Design review of the part built by this model. Coordinates are the model's own, in mm. A direction names the side the tool comes from. Coordinates: 2 decimals unless noted, no trailing zeros. Loops run counter-clockwise (first coordinate to the right, second up) from the corner with the lowest first, then second, coordinate; pieces in that order, holes last. Notation, with made-up numbers: M -4.75,17.5 L 16.25,17.5 A6 cw 16.25,28.5 Z; hole C 73,7.5 d8. An arc over 180 degrees is marked long. Answer as a JSON object with one key per item and string values. Group by question number.
1. Consider section B-B (x = 0). State the section outline as (y, z) points, then the cut area to 3 significant figures.
2. Consider section C-C (z = 0.5). State the section outline as (x, y) points, then the cut area to 3 significant figures.
3. Draft analysis for pull direction Y (two halves, no side actions). For faces 1 (the cylindrical face through (-0.867, -3.905, 4.085)), 2 (the flat face through (0, 0, 0)), 3 (the flat face through (1.748, 0.986, 6.028)), state which applies: +Y half, -Y half, draft (parallel to the pull), parting line (faces both ways), or undercut.
4. Insertion check: pin 1 (0.6 mm diameter, centred on x = 0.5, z = 5.5, fed in from -Y) (3 decimals); pin 2 (2 mm diameter, centred on x = 3, z = 6.5, fed in from -Y); pin 3 (4 mm diameter, centred on x = 2.5, z = 2.5, fed in from +Y). Each pin has a flat end and moves straight along its axis. Give the tip position at first contact, or say it passes through.
5. To check wall thickness, follow probe 1 along Y at (x, z) = (-2, 6); probe 2 along Z at (x, y) = (1.5, -1.25); probe 3 along Y at (x, z) = (1.75, 5.25). State the ranges of each line that lie inside material, in increasing order.
6. Consider section A-A (z = 5). State the section outline as (x, y) points.
7. Machinability: for faces 4 (the flat face through (-1.73, 1.01, 6.03)), 5 (the flat face through (2, 1, 8)), which of the approach directions +Z, -Z, +X, -X, +Y, -Y give a long, thin tool a straight path to every point of the face, cutting with its end or side? Answer none if there is none.
from build123d import *

# Parameters (mm, degrees)
ESQUISSE1_R             = 4
BASE_EXTRUSION_DEPTH    = 8
CHANFREIN1_SIZE         = 1.25
ENL_V_MAT_EXTRU_1_DEPTH = 4
CHANFREIN2_SIZE         = 1


with BuildPart() as part:
    # Esquisse1 → Base-Extrusion (new body)
    with BuildSketch(Plane.XY):
        Circle(ESQUISSE1_R)
    extrude(amount=BASE_EXTRUSION_DEPTH)

    # Chanfrein1
    chanfrein1_edges = [part.edges().sort_by_distance(p)[0] for p in [
        (-4, 0, 0),
    ]]
    chamfer(chanfrein1_edges, length=CHANFREIN1_SIZE)

    # Esquisse2 → Enlèv. mat.-Extru.1 (cut)
    with BuildSketch(Plane.XY.offset(8)):
        Polygon((2.415171399, 0), (1.061268564, 2), (-1.061268564, 2), (-2.415171399, 0), (-1.061268564, -2), (1.061268564, -2), align=None)
    extrude(amount=-ENL_V_MAT_EXTRU_1_DEPTH, mode=Mode.SUBTRACT)

    # Chanfrein2
    chanfrein2_edges = [part.edges().sort_by_distance(p)[0] for p in [
        (-4, 0, 8),
    ]]
    chamfer(chanfrein2_edges, length=CHANFREIN2_SIZE)


solid = part.part
Findings below:
{
 "1": {"outline": "M -4,1.25 L -2.75,0 L 2.75,0 L 4,1.25 L 4,7 L 3,8 L 2,8 L 2,4 L -2,4 L -2,8 L -3,8 L -4,7 Z", "area": "45.4 mm^2"},
 "2": {"outline": "C 0,0 d6.5", "area": "33.2 mm^2"},
 "3": {"face 1": "parting line", "face 2": "draft", "face 3": "undercut"},
 "4": {"pin 1": "stops at y = -3.995", "pin 2": "stops at y = -3.46", "pin 3": "stops at y = 3.97"},
 "5": {"probe 1": "y = -3.46 to -0.61, 0.61 to 3.46", "probe 2": "z = 0 to 4", "probe 3": "y = -3.6 to -0.98, 0.98 to 3.6"},
 "6": {"outline": "C 0,0 d8; hole M -2.42,0 L -1.06,-2 L 1.06,-2 L 2.42,0 L 1.06,2 L -1.06,2 Z"},
 "7": {"face 4": "+Z", "face 5": "+Z, +X, -X, +Y, -Y"}
}
